```python
from build123d import *

# Parameters (mm, degrees)
F0_W     = 81
F0_H     = 44
F1_DEPTH = 2
F2_DEPTH = 5
F3_R     = 1


with BuildPart() as f1:
    # F0 (on Top) → F1 (new body)
    with BuildSketch(Plane.XY):
        with BuildLine():
            Line((-41, -25.5), (41, -25.5))
            ThreePointArc((41, -25.5), (43.1213203436, -24.6213203436), (44, -22.5))
            Line((44, -22.5), (44, 22.5))
            ThreePointArc((44, 22.5), (43.1213203436, 24.6213203436), (41, 25.5))
            Line((41, 25.5), (-41, 25.5))
            ThreePointArc((-41, 25.5), (-43.1213203436, 24.6213203436), (-44, 22.5))
            Line((-44, 22.5), (-44, -22.5))
            ThreePointArc((-44, -22.5), (-43.1213203436, -24.6213203436), (-41, -25.5))
        make_face()
        with BuildLine():
            Line((-40, 23.5), (40, 23.5))
            ThreePointArc((40, 23.5), (41.4142135624, 22.9142135624), (42, 21.5))
            Line((42, 21.5), (42, -21.5))
            ThreePointArc((42, -21.5), (41.4142135624, -22.9142135624), (40, -23.5))
            Line((40, -23.5), (-40, -23.5))
            ThreePointArc((-40, -23.5), (-41.4142135624, -22.9142135624), (-42, -21.5))
            Line((-42, -21.5), (-42, 21.5))
            ThreePointArc((-42, 21.5), (-41.4142135624, 22.9142135624), (-40, 23.5))
        make_face(mode=Mode.SUBTRACT)
        with BuildLine():
            ThreePointArc((42, 21.5), (41.4142135624, 22.9142135624), (40, 23.5))
            Line((40, 23.5), (-40, 23.5))
            ThreePointArc((-40, 23.5), (-41.4142135624, 22.9142135624), (-42, 21.5))
            Line((-42, 21.5), (-42, -21.5))
            ThreePointArc((-42, -21.5), (-41.4142135624, -22.9142135624), (-40, -23.5))
            Line((-40, -23.5), (40, -23.5))
            ThreePointArc((40, -23.5), (41.4142135624, -22.9142135624), (42, -21.5))
            Line((42, -21.5), (42, 21.5))
        make_face()
        Rectangle(F0_W, F0_H, mode=Mode.SUBTRACT)
        Rectangle(F0_W, F0_H)
    extrude(amount=F1_DEPTH)

    # F0 (on Top) → F2 (join)
    with BuildSketch(Plane.XY):
        with BuildLine():
            ThreePointArc((42, 21.5), (41.4142135624, 22.9142135624), (40, 23.5))
            Line((40, 23.5), (-40, 23.5))
            ThreePointArc((-40, 23.5), (-41.4142135624, 22.9142135624), (-42, 21.5))
            Line((-42, 21.5), (-42, -21.5))
            ThreePointArc((-42, -21.5), (-41.4142135624, -22.9142135624), (-40, -23.5))
            Line((-40, -23.5), (40, -23.5))
            ThreePointArc((40, -23.5), (41.4142135624, -22.9142135624), (42, -21.5))
            Line((42, -21.5), (42, 21.5))
        make_face()
        Rectangle(F0_W, F0_H, mode=Mode.SUBTRACT)
    extrude(amount=F2_DEPTH)

    # F3
    f3_edges = [f1.edges().sort_by_distance(p)[0] for p in [
        (-42, 0, 5),
    ]]
    fillet(f3_edges, radius=F3_R)


solid = f1.part
```
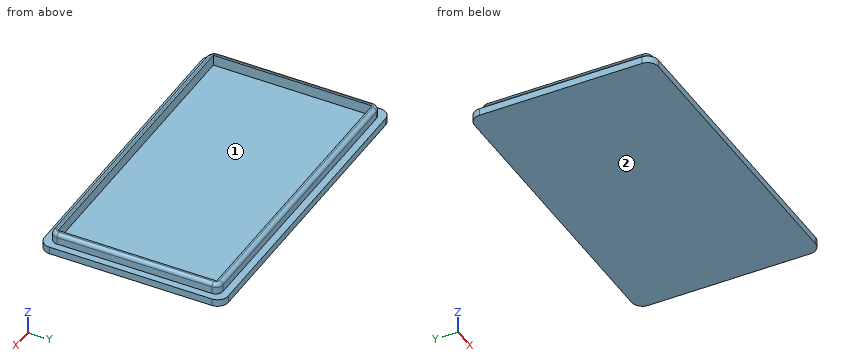
The listing builds one solid part. Answer for the finished solid, in the listing's coordinates (mm). Face numbers are marked on the shaded views. Give positions to 0.01 mm unless a question says otherwise; leave off trailing zeros. Order: outer loops, then holes, each group sorted by start corner. A loop starts at its lowest first (then second) coordinate and runs counter-clockwise, first axis right, second up. Notation, with made-up numbers: (25.5, 27) - (76.5, 27) arc R12 ccw to (76.5, 37) - close; hole circle Ø4 at (-17, 39). An arc over 180 degrees is marked (long way). Use one line per item in the form item = value. Start each with the question number.
(1) The mould has two halves that part along X. Classify the marked faces 1 and 2: released by +X, released by -X, zero draft, split by the parting line, or undercut.
(2) A cutting plane is placed at A-A, the plane y = -5. Write down the section's boundary in (x, z), then the cut area to 3 significant figures.
(3) A cutting plane is placed at B-B, the plane x = -18.5. Write down the section's boundary in (y, z), then the cut area to 3 significant figures.
(4) Consider line 1 (Y direction, x = -7, z = 2.4); line 2 (X direction, y = -10.5, z = 3.25); line 3 (Z direction, x = -0.5, y = -20.5). Determine where each line is inside the solid, lowest interval first. Write a range as from..to.
(5) Flat-ended cylindrical pins translate along their axes: pin 1 Ø0.6 at (x, z) = (9.5, 2.5) entering from -Y; pin 2 Ø2.5 at (x, z) = (6.5, 4) entering from +Y; pin 3 Ø5 at (x, y) = (5, 6) entering from +Z; pin 4 Ø10 at (x, y) = (-30, -19.5) entering from -Z. Find the tip coordinate at first contact, or state that the pin passes through.
Ans:
q1.face_1 = undercut
q1.face_2 = zero draft
q2.outline = (-44, 0) - (44, 0) - (44, 2) - (42, 2) - (42, 4) arc R1 ccw to (41, 5) - (40.5, 5) - (40.5, 2) - (-40.5, 2) - (-40.5, 5) - (-41, 5) arc R1 ccw to (-42, 4) - (-42, 2) - (-44, 2) - close
q2.area = 185 mm^2
q3.outline = (-25.5, 0) - (25.5, 0) - (25.5, 2) - (23.5, 2) - (23.5, 4) arc R1 ccw to (22.5, 5) - (22, 5) - (22, 2) - (-22, 2) - (-22, 5) - (-22.5, 5) arc R1 ccw to (-23.5, 4) - (-23.5, 2) - (-25.5, 2) - close
q3.area = 111 mm^2
q4.line_1 = -23.5..-22, 22..23.5
q4.line_2 = -42..-40.5, 40.5..42
q4.line_3 = 0..2
q5.pin_1 = -23.5
q5.pin_2 = 23.5
q5.pin_3 = 2
q5.pin_4 = 0
